Check sheet for the drawn part. Datum: minimum x, y, z corner. Units: mm. A direction names the side the tool comes from. Round coordinates to 2 decimals unless told otherwise and drop trailing zeros. Write each loop counter-clockwise with the first axis right and the second up, starting at its lowest first coordinate (ties: lowest second). Pieces come first, ordered by that corner, then holes.
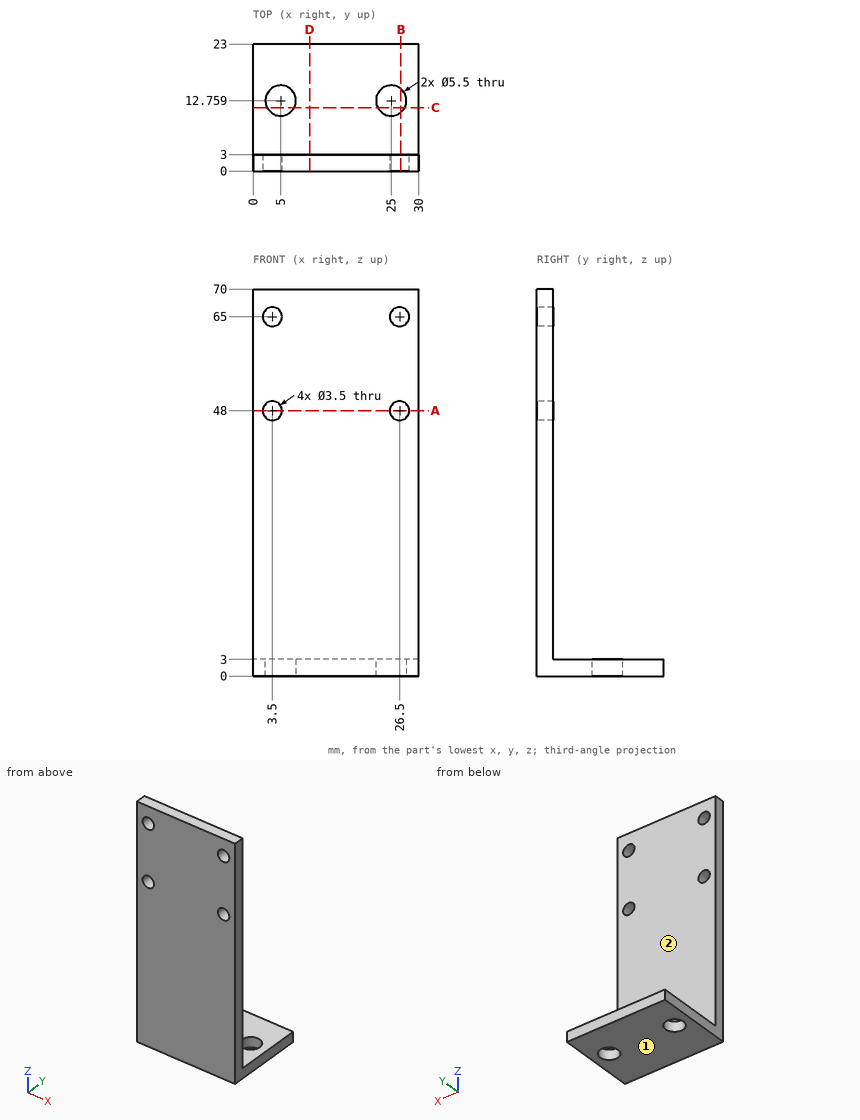
Q1. Sectioned sample at D-D (x = 10.25). Enter the section's corners in (y, z), plus the area to 3 significant figures.
Recorded:
outline: (0, 0) - (23, 0) - (23, 3) - (3, 3) - (3, 70) - (0, 70) - close
area: 270 mm2
Q2. Depth check by flat-ended pin: P1, Ø2, axis at x = 3.5, z = 48, coming from the -Y side; P2, Ø4, axis at x = 26.5, z = 48, coming from the +Y side; P3, Ø1.5, axis at x = 5.5, y = 16, coming from the +Z side. Enter the tip coordinate at first touch or a pass-through.
Recorded:
P1: passes through
P2: stops at y = 3
P3: stops at z = 3
Q3. Material ranges on line 1 along X through (y, z) = (2.05, 65); line 2 along Z through (x, y) = (3.5, 1.9); line 3 along Y through (x, z) = (5, 1.8), recorded low to high.
Recorded:
line 1: x = 0 to 1.75, 5.25 to 24.75, 28.25 to 30
line 2: z = 0 to 46.25, 49.75 to 63.25, 66.75 to 70
line 3: y = 0 to 10.01, 15.51 to 23
Q4. Sectioned sample at C-C (y = 11.5). Enter the section's corners in (x, z) (3 decimals).
Recorded:
outline: (0, 0) - (2.555, 0) - (2.555, 3) - (0, 3) - close; (7.445, 0) - (22.555, 0) - (22.555, 3) - (7.445, 3) - close; (27.445, 0) - (30, 0) - (30, 3) - (27.445, 3) - close
Q5. Tool access check on the marked faces 1 and 2. Record the directions out of +Z, -Z, +X, -X, +Y, -Y that give a thin tool (end or side, any length) a straight path to the whole face; none if there is none.
Recorded:
face 1: -Z, +X, -X, +Y, -Y
face 2: +Z, +X, -X, +Y
Q6. Sectioned sample at A-A (z = 48). Enter the section's corners in (x, y), plus the area to 3 significant figures.
Recorded:
outline: (0, 0) - (1.75, 0) - (1.75, 3) - (0, 3) - close; (5.25, 0) - (24.75, 0) - (24.75, 3) - (5.25, 3) - close; (28.25, 0) - (30, 0) - (30, 3) - (28.25, 3) - close
area: 69.0 mm2
Q7. Sectioned sample at B-B (x = 26.75). Enter the section's corners in (y, z).
Recorded:
outline: (0, 0) - (10.64, 0) - (10.64, 3) - (3, 3) - (3, 46.27) - (0, 46.27) - close; (0, 49.73) - (3, 49.73) - (3, 63.27) - (0, 63.27) - close; (0, 66.73) - (3, 66.73) - (3, 70) - (0, 70) - close; (14.88, 0) - (23, 0) - (23, 3) - (14.88, 3) - close
